Design review of the part built by this model. Coordinates are the model's own, in mm. Coordinates: 2 decimals unless noted, no trailing zeros. Loops run counter-clockwise (first coordinate to the right, second up) from the corner with the lowest first, then second, coordinate; pieces in that order, holes last. Notation, with made-up numbers: (-30, 57) -> (-3, 57) arc R26 cw to (-3, 76) -> close; hole circle Ø7 at (-20.5, 71). An arc over 180 degrees is marked (long way). Use one line per item in the form item = value. Start each with the question number.
1. Wall thickness on line 1 (Z direction, x = 21.5, y = 9); line 2 (Z direction, x = 19, y = 3.5); line 3 (Y direction, x = 24, z = 27): over which ranges is each line inside the solid? List them lowest first. Write a range as from..to.
2. For pin 1 (12 mm diameter, centred on y = 19.5, z = 7.5, fed in from +X); pin 2 (1 mm diameter, centred on y = 8, z = 41.5, fed in from +X); pin 3 (2 mm diameter, centred on x = 10.5, z = 14.5, fed in from -Y), all flat-tipped, find the tip position at first contact; note any pin that passes through.
3. Consider section A-A (z = 38). State the section outline as (x, y) points.
4. The part is to be moulded in two halves that separate along X. For faces 1 (the face through (12, 17, 50.8)), 2 (the face through (0.98, 34.69, 25.43)), 3 (the face through (29.225, 0.421, 25.747)), 4 (the face through (26.16, 2.79, 25.43)), say which applies: released by +X, released by -X, zero draft, split by the parting line, or undercut.
from build123d import *

# Parameters (mm, degrees)
F1_DEPTH     = 50.8
F2_W         = 48.4209248795
F2_H         = 50.8
F2_W_2       = 40.64
F2_H_2       = 40.64
F3_DEPTH     = 7.62
F4_T1_DEPTH  = 40.64
F4_T3_DEPTH  = 40.64
F4_T9_DEPTH  = 53.34
F4_T15_DEPTH = 53.34
F4_T24_DEPTH = 53.34
F4_T30_DEPTH = 53.34
F5_T1_DEPTH  = 40.64
F5_T6_DEPTH  = 17.2700101558
F5_S7_R      = 5.0800000001
F5_T8_DEPTH  = 13
F5_T12_DEPTH = 15.9109147238
F5_S13_R     = 5.0800000001
F5_T14_DEPTH = 12
F6_R         = 5.08


# Not quite as in the source:
# - a fillet or chamfer that OpenCascade refuses, or shapes differently, is made with other operations: its cross-section is extruded or revolved along the edge and cut away or added


with BuildPart() as f1:
    # F0 (on Top) → F1 (new body)
    with BuildSketch(Plane.XY):
        with BuildLine():
            Line((0, 38.0047485232), (30.0037506968, 0))
            ThreePointArc((30.0037506968, 0), (19.9032134253, 22.871851931), (0, 38.0047485232))
        make_face()
    extrude(amount=F1_DEPTH)

    # F2 (on face) → F3 (join)
    with BuildSketch(Plane(origin=(18.4835383706, 14.5922680406, 0), x_dir=(0.6196443123, -0.7848827468, 0), z_dir=(-0.7848827468, -0.6196443123, 0))):
        with Locations((-5.6188089735, 25.4)):
            Rectangle(F2_W, F2_H)
        with Locations((-6.2983566895, 25.7165116596)):
            Rectangle(F2_W_2, F2_H_2, mode=Mode.SUBTRACT)
    extrude(amount=F3_DEPTH)

    # F4: fillet of radius 5.08 on 3 edges, made by hand

    # F4_s2 → F4_t1 (cut)
    with BuildSketch(Plane(origin=(-16.4939133248, 20.8922889144, 0), x_dir=(0, 0, 1), z_dir=(0.6196443123, -0.7848827468, 0))):
        with BuildLine():
            ThreePointArc((46.0365116596, -21.0094262619), (47.5244092112, -17.4173238135), (51.1165116596, -15.9294262619))
            Line((51.1165116596, -15.9294262619), (46.0365116596, -15.9294262619))
            Line((46.0365116596, -15.9294262619), (46.0365116596, -21.0094262619))
        make_face()
    extrude(amount=F4_T1_DEPTH, mode=Mode.SUBTRACT)

    # F4_s4 → F4_t3 (cut)
    with BuildSketch(Plane.XY.offset(5.3965116596)):
        with BuildLine():
            ThreePointArc((25.1783677198, 2.0130255709), (23.2809557383, -1.3806253977), (24.3389564723, -5.1219718894))
            Line((24.3389564723, -5.1219718894), (21.1911633659, -1.1347675355))
            Line((21.1911633659, -1.1347675355), (25.1783677198, 2.0130255709))
        make_face()
        with BuildLine():
            ThreePointArc((-0.0039771311, 33.9106604018), (-3.7453236228, 32.8526596678), (-7.1389745914, 34.7500716493))
            Line((-7.1389745914, 34.7500716493), (-3.991181485, 30.7628672955))
            Line((-3.991181485, 30.7628672955), (-0.0039771311, 33.9106604018))
        make_face()
    extrude(amount=F4_T3_DEPTH, mode=Mode.SUBTRACT)


with BuildPart() as f4_tool7:
    # F4_s8 → F4_t9 (new body)
    with BuildSketch(Plane(origin=(-24.3633960907, 30.8602997991, 0), x_dir=(0, 0, 1), z_dir=(0.6196443123, -0.7848827468, 0))):
        with BuildLine():
            ThreePointArc((46.0365116596, -21.0094262619), (47.5244092112, -17.4173238135), (51.1165116596, -15.9294262619))
            Line((51.1165116596, -15.9294262619), (46.0365116596, -15.9294262619))
            Line((46.0365116596, -15.9294262619), (46.0365116596, -21.0094262619))
        make_face()
    extrude(amount=F4_T9_DEPTH)

    split(bisect_by=Plane(origin=(-16.4939133248, 20.8922889144, 0), x_dir=(0, 0, 1), z_dir=(-0.6196443123, 0.7848827468, 0)), keep=Keep.TOP)

    split(bisect_by=Plane.XY.offset(50.8), keep=Keep.BOTTOM)

    split(bisect_by=Plane(origin=(-18.4835383706, 23.4124804826, 0), x_dir=(0, 0, 1), z_dir=(0.6196443123, -0.7848827468, 0)), keep=Keep.TOP)


with BuildPart() as f4_tool13:
    # F4_s14 → F4_t15 (new body)
    with BuildSketch(Plane.XY.offset(5.3965116596)):
        with BuildLine():
            ThreePointArc((-0.0039771311, 33.9106604018), (-3.7453236228, 32.8526596678), (-7.1389745914, 34.7500716493))
            Line((-7.1389745914, 34.7500716493), (-3.991181485, 30.7628672955))
            Line((-3.991181485, 30.7628672955), (-0.0039771311, 33.9106604018))
        make_face()
    extrude(amount=F4_T15_DEPTH)

    split(bisect_by=Plane.XY.offset(46.0365116596), keep=Keep.TOP)

    split(bisect_by=Plane.XY.offset(50.8), keep=Keep.BOTTOM)

    split(bisect_by=Plane(origin=(-18.4835383706, 23.4124804826, 0), x_dir=(0, 0, 1), z_dir=(0.6196443123, -0.7848827468, 0)), keep=Keep.TOP)


with BuildPart() as f4_tool7_1:
    add(f4_tool7.part)

    # F4_t19: intersect F4_tool13
    add(f4_tool13.part, mode=Mode.INTERSECT)


with BuildPart() as f1_1:
    add(f1.part)

    # F4_t5: cut F4_tool7
    add(f4_tool7_1.part, mode=Mode.SUBTRACT)


with BuildPart() as f4_tool22:
    # F4_s23 → F4_t24 (new body)
    with BuildSketch(Plane(origin=(-16.4939133248, 20.8922889144, 0), x_dir=(0, 0, 1), z_dir=(0.6196443123, -0.7848827468, 0))):
        with BuildLine():
            ThreePointArc((46.0365116596, -21.0094262619), (47.5244092112, -17.4173238135), (51.1165116596, -15.9294262619))
            Line((51.1165116596, -15.9294262619), (46.0365116596, -15.9294262619))
            Line((46.0365116596, -15.9294262619), (46.0365116596, -21.0094262619))
        make_face()
    extrude(amount=F4_T24_DEPTH)

    split(bisect_by=Plane(origin=(8.6884315261, -11.0053459165, 0), x_dir=(0, 0, 1), z_dir=(0.6196443123, -0.7848827468, 0)), keep=Keep.TOP)

    split(bisect_by=Plane(origin=(11.5202123262, -14.5922680406, 0), x_dir=(0, 0, 1), z_dir=(-0.6196443123, 0.7848827468, 0)), keep=Keep.TOP)

    split(bisect_by=Plane.XY.offset(50.8), keep=Keep.BOTTOM)


with BuildPart() as f4_tool28:
    # F4_s29 → F4_t30 (new body)
    with BuildSketch(Plane.XY.offset(58.7365116596)):
        with BuildLine():
            ThreePointArc((25.1783677198, 2.0130255709), (23.2809557383, -1.3806253977), (24.3389564723, -5.1219718894))
            Line((24.3389564723, -5.1219718894), (21.1911633659, -1.1347675355))
            Line((21.1911633659, -1.1347675355), (25.1783677198, 2.0130255709))
        make_face()
    extrude(amount=-F4_T30_DEPTH)

    split(bisect_by=Plane.XY.offset(46.0365116596), keep=Keep.TOP)

    split(bisect_by=Plane(origin=(11.5202123262, -14.5922680406, 0), x_dir=(0, 0, 1), z_dir=(-0.6196443123, 0.7848827468, 0)), keep=Keep.TOP)

    split(bisect_by=Plane.XY.offset(50.8), keep=Keep.BOTTOM)


with BuildPart() as f4_tool22_1:
    add(f4_tool22.part)

    # F4_t34: intersect F4_tool28
    add(f4_tool28.part, mode=Mode.INTERSECT)


with BuildPart() as f1_2:
    add(f1_1.part)

    # F4_t20: cut F4_tool22
    add(f4_tool22_1.part, mode=Mode.SUBTRACT)

    # F5: fillet of radius 5.08 on 1 edges, made by hand

    # F5_s2 → F5_t1 (cut)
    with BuildSketch(Plane(origin=(8.6884315261, -11.0053459165, 0), x_dir=(0, 0, 1), z_dir=(-0.6196443123, 0.7848827468, 0))):
        with BuildLine():
            ThreePointArc((0.3165116596, 15.9294262619), (3.908614108, 17.4173238135), (5.3965116596, 21.0094262619))
            Line((5.3965116596, 21.0094262619), (5.3965116596, 15.9294262619))
            Line((5.3965116596, 15.9294262619), (0.3165116596, 15.9294262619))
        make_face()
    extrude(amount=F5_T1_DEPTH, mode=Mode.SUBTRACT)


with BuildPart() as f5_tool4:
    # F5_s5 → F5_t6 (new body)
    with BuildSketch(Plane(origin=(19.3896950922, -24.5602789253, 0), x_dir=(0, 0, 1), z_dir=(-0.6196443123, 0.7848827468, 0))):
        with BuildLine():
            ThreePointArc((0.3165116596, 15.9294262619), (3.908614108, 17.4173238135), (5.3965116596, 21.0094262619))
            Line((5.3965116596, 21.0094262619), (5.3965116596, 15.9294262619))
            Line((5.3965116596, 15.9294262619), (0.3165116596, 15.9294262619))
        make_face()
    extrude(amount=F5_T6_DEPTH)

    # F5_s7 → F5_t8 (cut, symmetric)
    with BuildSketch(Plane.XY.offset(2.9)):
        with Locations((28.3261608263, -1.974178783)):
            Circle(F5_S7_R)
    extrude(amount=F5_T8_DEPTH, both=True, mode=Mode.SUBTRACT)


with BuildPart() as f1_3:
    add(f1_2.part)

    # F5_t3: cut F5_tool4
    add(f5_tool4.part, mode=Mode.SUBTRACT)


with BuildPart() as f5_tool10:
    # F5_s11 → F5_t12 (new body)
    with BuildSketch(Plane(origin=(-26.3530211368, 33.3804913668, 0), x_dir=(0, 0, 1), z_dir=(0.6196443123, -0.7848827468, 0))):
        with BuildLine():
            ThreePointArc((0.3165116596, -15.9294262623), (3.908614108, -17.4173238139), (5.3965116596, -21.0094262623))
            Line((5.3965116596, -21.0094262623), (5.3965116596, -15.9294262623))
            Line((5.3965116596, -15.9294262623), (0.3165116596, -15.9294262623))
        make_face()
    extrude(amount=F5_T12_DEPTH)

    # F5_s13 → F5_t14 (cut, symmetric)
    with BuildSketch(Plane.XY.offset(2.9)):
        with Locations((-3.1517702375, 37.8978647558)):
            Circle(F5_S13_R)
    extrude(amount=F5_T14_DEPTH, both=True, mode=Mode.SUBTRACT)


with BuildPart() as f1_4:
    add(f1_3.part)

    # F5_t9: cut F5_tool10
    add(f5_tool10.part, mode=Mode.SUBTRACT)

    # F6
    f6_edges = [f1_4.edges().sort_by_distance(p)[0] for p in [
        (19.903213, 22.871852, 50.8),
        (30.003751, 0, 25.4),
        (19.903213, 22.871852, 0),
        (0, 38.004749, 25.4),
    ]]
    fillet(f6_edges, radius=F6_R)


solid = f1_4.part
Geometry check:
q1.line_1 = 0..5.4, 46.04..50.8
q1.line_2 = 0..3.54, 47.9..50.8
q1.line_3 = -4.64..0.69, 7.6..16.82
q2.pin_1 = 25.75
q2.pin_2 = 28.16
q2.pin_3 = 23.44
q3.outline = (-5.7, 33.5) arc R5.08 ccw to (0, 33.91) -> (1.99, 35.48) -> (27.17, 3.59) -> (25.18, 2.01) arc R5.08 ccw to (24.04, -4.71) -> (27.57, -1.93) arc R5.08 ccw to (29.36, 3.21) arc R50.05 ccw to (2.98, 36.64) arc R5.08 ccw to (-2.44, 36.08) -> close
q4.face_1 = zero draft
q4.face_2 = undercut
q4.face_3 = released by +X
q4.face_4 = released by -X
